The listing builds one solid part. Answer for the finished solid, in the listing's coordinates (mm). A direction names the side the tool comes from. Give positions to 0.01 mm unless a question says otherwise; leave off trailing zeros. Loops run counter-clockwise (first coordinate to the right, second up) from the corner with the lowest first, then second, coordinate; pieces in that order, holes last. Notation, with made-up numbers: (31, -12) - (48, -12) arc R34 cw to (48, 26) - close; hole circle Ø5 at (6.5, -15.5). An arc over 180 degrees is marked (long way). Write item = value, one per line. Start each with the question number.
1) The part is cut by section B-B on y = 36. Write down the section's boundary in (x, z).
2) The part is cut by section C-C on x = 4.5. Write down the section's boundary in (y, z).
3) Consider probe 1 along X at (y, z) = (17, 2.45); probe 2 along Y at (x, z) = (4, 0.6); probe 3 along Y at (x, z) = (-14, 2.6). Determine where each line is inside the solid, lowest interval first.
4) The part is cut by section A-A on x = 14. Write down the section's boundary in (y, z).
5) Which of the six approach directions +Z, -Z, +X, -X, +Y, -Y give full straight-line access (tool end or side, diameter ignored) to faces 1 (the flat face through (1, 11.002, 2)), 2 (the flat face through (-26.679, 18, 2)), 3 (the flat face through (-22.949, 55, 2))?
6) The part is cut by section D-D on y = -19.5. Write down the section's boundary in (x, z).
7) Flat-ended cylindrical pins translate along their axes: P1, Ø1.2, axis at y = 10, z = 2.5, coming from the -X side; P2, Ø1.6, axis at y = -10.5, z = 3, coming from the -X side. Find the tip coordinate at first contact, or state that the pin passes through.
from build123d import *

# Parameters (mm, degrees)
SKETCH1_R           = 1.75
SKETCH1_R_2         = 2.15
SKETCH1_W           = 15
SKETCH1_H           = 2.7
BOSS_EXTRUDE1_DEPTH = 5


with BuildPart() as part:
    # Sketch1 → Boss-Extrude1 (new body)
    with BuildSketch(Plane.XY):
        with BuildLine():
            Line((33.050798555, 66.930419372), (-18.949201445, 66.930419372))
            ThreePointArc((-18.949201445, 66.930419372), (-21.77762857, 65.758846497), (-22.949201445, 62.930419372))
            Line((-22.949201445, 62.930419372), (-22.949201445, 45.959184597))
            add(Edge.make_bspline(
                [(-26.015204316, 44.603739403), (-25.073035607, 45.327145808), (-24.05103465, 45.778960873), (-22.949201445, 45.959184597)],
                knots=[0, 0, 0, 0, 0.632660701, 0.632660701, 0.632660701, 0.632660701], degree=3))
            ThreePointArc((-26.015204316, 44.603739403), (-27.948018841, 43.367577553), (-28.7, 41.2))
            Line((-28.7, 41.2), (-28.7, 28.8))
            ThreePointArc((-28.7, 28.8), (-28.151687317, 26.919164552), (-26.678547439, 25.62763535))
            Line((-26.678547439, 25.62763535), (-26.678547439, 9.37236465))
            ThreePointArc((-26.678547439, 9.37236465), (-28.151687317, 8.080835448), (-28.7, 6.2))
            Line((-28.7, 6.2), (-28.7, -6.2))
            ThreePointArc((-28.7, -6.2), (-27.948018841, -8.367577553), (-26.015204316, -9.603739403))
            add(Edge.make_bspline(
                [(-26.015204316, -9.603739403), (-25.073035607, -10.327145808), (-24.05103465, -10.778960873), (-22.949201445, -10.959184597)],
                knots=[0, 0, 0, 0, 0.632660701, 0.632660701, 0.632660701, 0.632660701], degree=3))
            Line((-22.949201445, -10.959184597), (-22.949201445, -30.315366628))
            ThreePointArc((-22.949201445, -30.315366628), (-21.77762857, -33.143793753), (-18.949201445, -34.315366628))
            Line((-18.949201445, -34.315366628), (33.050798555, -34.315366628))
            ThreePointArc((33.050798555, -34.315366628), (35.879225679, -33.143793753), (37.050798555, -30.315366628))
            Line((37.050798555, -30.315366628), (37.050798555, 62.930419372))
            ThreePointArc((37.050798555, 62.930419372), (35.879225679, 65.758846497), (33.050798555, 66.930419372))
        make_face()
        with Locations((-25.2, -6.2)):
            Circle(SKETCH1_R, mode=Mode.SUBTRACT)
        with Locations((-25.2, 6.2)):
            Circle(SKETCH1_R, mode=Mode.SUBTRACT)
        with Locations((-17.949201445, 61.930418903)):
            Circle(SKETCH1_R_2, mode=Mode.SUBTRACT)
        with Locations((32.050798555, 61.930418903)):
            Circle(SKETCH1_R_2, mode=Mode.SUBTRACT)
        with Locations((32.050798555, -29.315366628)):
            Circle(SKETCH1_R_2, mode=Mode.SUBTRACT)
        with Locations((-17.949201445, -29.315366628)):
            Circle(SKETCH1_R_2, mode=Mode.SUBTRACT)
        with Locations((25.2, 28.8)):
            Circle(SKETCH1_R, mode=Mode.SUBTRACT)
        with Locations((25.2, 41.2)):
            Circle(SKETCH1_R, mode=Mode.SUBTRACT)
        with Locations((-25.2, 28.8)):
            Circle(SKETCH1_R, mode=Mode.SUBTRACT)
        with Locations((-25.2, 41.2)):
            Circle(SKETCH1_R, mode=Mode.SUBTRACT)
        with Locations((25.2, 6.2)):
            Circle(SKETCH1_R, mode=Mode.SUBTRACT)
        with Locations((25.2, -6.2)):
            Circle(SKETCH1_R, mode=Mode.SUBTRACT)
        with BuildLine():
            Line((-20.949201445, 46.122161619), (24.050798555, 46.122161619))
            Line((24.050798555, 46.122161619), (24.050798555, 44.505954633))
            ThreePointArc((24.050798555, 44.505954633), (21.732055874, 41.672613518), (23.208062077, 38.322121735))
            Line((23.208062077, 38.322121735), (23.208062077, 31.677878265))
            ThreePointArc((23.208062077, 31.677878265), (21.732055874, 28.327386482), (24.050798555, 25.494045367))
            Line((24.050798555, 25.494045367), (24.050798555, 24.122161619))
            Line((24.050798555, 24.122161619), (-20.949201445, 24.122161619))
            Line((-20.949201445, 24.122161619), (-20.949201445, 46.122161619))
        make_face(mode=Mode.SUBTRACT)
        with BuildLine():
            Line((-20.949201445, 11.001569649), (24.050798555, 11.001569649))
            Line((24.050798555, 11.001569649), (24.050798555, 9.505954633))
            ThreePointArc((24.050798555, 9.505954633), (21.732055874, 6.672613518), (23.208062077, 3.322121735))
            Line((23.208062077, 3.322121735), (23.208062077, -3.322121735))
            ThreePointArc((23.208062077, -3.322121735), (21.732055874, -6.672613518), (24.050798555, -9.505954633))
            Line((24.050798555, -9.505954633), (24.050798555, -10.998430351))
            Line((24.050798555, -10.998430351), (-20.949201445, -10.998430351))
            Line((-20.949201445, -10.998430351), (-20.949201445, 11.001569649))
        make_face(mode=Mode.SUBTRACT)
        with Locations((-11.449201445, 17.5)):
            Rectangle(SKETCH1_W, SKETCH1_H, mode=Mode.SUBTRACT)
        with Locations((18.550798555, 17.5)):
            Rectangle(SKETCH1_W, SKETCH1_H, mode=Mode.SUBTRACT)
    extrude(amount=BOSS_EXTRUDE1_DEPTH)


solid = part.part
Answer below:
q1.outline = (-28.7, 0) - (-20.95, 0) - (-20.95, 5) - (-28.7, 5) - close; (23.21, 0) - (37.05, 0) - (37.05, 5) - (23.21, 5) - close
q2.outline = (-34.32, 0) - (-11, 0) - (-11, 5) - (-34.32, 5) - close; (11, 0) - (24.12, 0) - (24.12, 5) - (11, 5) - close; (46.12, 0) - (66.93, 0) - (66.93, 5) - (46.12, 5) - close
q3.probe_1 = -26.68 to -18.95, -3.95 to 11.05, 26.05 to 37.05
q3.probe_2 = -34.32 to -11, 11 to 24.12, 46.12 to 66.93
q3.probe_3 = -34.32 to -11, 11 to 16.15, 18.85 to 24.12, 46.12 to 66.93
q4.outline = (-34.32, 0) - (-11, 0) - (-11, 5) - (-34.32, 5) - close; (11, 0) - (16.15, 0) - (16.15, 5) - (11, 5) - close; (18.85, 0) - (24.12, 0) - (24.12, 5) - (18.85, 5) - close; (46.12, 0) - (66.93, 0) - (66.93, 5) - (46.12, 5) - close
q5.face_1 = +Z, -Z
q5.face_2 = +Z, -Z, -X
q5.face_3 = +Z, -Z, -X, +Y
q6.outline = (-22.95, 0) - (37.05, 0) - (37.05, 5) - (-22.95, 5) - close
q7.P1 = -26.68
q7.P2 = -25.89
